```python
from build123d import *

# Parameters (mm, degrees)
SKETCH1_W           = 10
SKETCH1_H           = 7
BOSS_EXTRUDE1_DEPTH = 2
SKETCH2_R           = 1.425
CUT_EXTRUDE1_DEPTH  = 2
SKETCH3_W           = 6
SKETCH3_H           = 1
BOSS_EXTRUDE2_DEPTH = 6


with BuildPart() as part:
    # Sketch1 → Boss-Extrude1 (new body)
    with BuildSketch(Plane(origin=(0, 0, 0), x_dir=(1, 0, 0), z_dir=(0, 1, 0))):
        Rectangle(SKETCH1_W, SKETCH1_H)
    extrude(amount=BOSS_EXTRUDE1_DEPTH)

    # Sketch2 → Cut-Extrude1 (cut)
    with BuildSketch(Plane(origin=(0, 2, 0), x_dir=(1, 0, 0), z_dir=(0, 1, 0))):
        Circle(SKETCH2_R)
    extrude(amount=-CUT_EXTRUDE1_DEPTH, mode=Mode.SUBTRACT)

    # Sketch3 → Boss-Extrude2 (add)
    with BuildSketch(Plane(origin=(0, 2, 0), x_dir=(1, 0, 0), z_dir=(0, 1, 0))):
        with Locations((0, -3)):
            Rectangle(SKETCH3_W, SKETCH3_H)
    boss_extrude2 = extrude(amount=BOSS_EXTRUDE2_DEPTH)

    # Mirror1: Boss-Extrude2 across plane
    add(boss_extrude2.mirror(Plane.XY))


solid = part.part
```
The listing builds one solid part. Answer for the finished solid, in the listing's coordinates (mm). A direction names the side the tool comes from. Give positions to 0.01 mm unless a question says otherwise; leave off trailing zeros. Order: outer loops, then holes, each group sorted by start corner. A loop starts at its lowest first (then second) coordinate and runs counter-clockwise, first axis right, second up.
Item 1: Given pin 1 Ø1.1 at (y, z) = (5.5, -3) entering from -X; pin 2 Ø2 at (y, z) = (5, 0.5) entering from +X, each flat-ended and moving along its own axis, determine where each tip first touches the part or whether it passes through.
From the geometry:
pin 1: stops at x = -3
pin 2: passes through
Item 2: For a pull along Z with two mould halves and no side action, classify faces 1 (the face through (0, 3, 3.5)), 2 (the face through (0, 5, -2.5)), 3 (the face through (0, 8, -3)) as pulls with the +Z half, pulls with the -Z half, needs draft (parallel to the pull), parting line crosses it, or undercut.
From the geometry:
face 1: pulls with the +Z half
face 2: undercut
face 3: needs draft
Item 3: The part is cut by section D-D, the plane y = 1.5. Give the vertices of the cut face in (x, z) (3 decimals).
From the geometry:
outline: (-5, -3.5) - (5, -3.5) - (5, 3.5) - (-5, 3.5) - close; hole circle Ø2.85 at (0, 0)
Item 4: Find the intervals of material crossed by probe 1 along Z at (x, y) = (0, 1.35) (3 decimals); probe 2 along X at (y, z) = (1.5, 0) (3 decimals); probe 3 along Z at (x, y) = (0, 5), in increasing order.
From the geometry:
probe 1: z = -3.5 to -1.425, 1.425 to 3.5
probe 2: x = -5 to -1.425, 1.425 to 5
probe 3: z = -3.5 to -2.5, 2.5 to 3.5
Item 5: Which of the six approach directions +Z, -Z, +X, -X, +Y, -Y give full straight-line access (tool end or side, diameter ignored) to faces 4 (the face through (-3, 5, 3)), 5 (the face through (0, 3, -3.5)), 6 (the face through (0, 5, 2.5)), 7 (the face through (3, 5, -3)), 8 (the face through (0, 8, 3))?
From the geometry:
face 4: +Z, -Z, -X, +Y
face 5: -Z, +X, -X, +Y, -Y
face 6: +X, -X, +Y
face 7: +Z, -Z, +X, +Y
face 8: +Z, -Z, +X, -X, +Y
Item 6: The part is cut by section A-A, the plane y = 5.25. Give the vertices of the cut face in (x, z).
From the geometry:
outline: (-3, -3.5) - (3, -3.5) - (3, -2.5) - (-3, -2.5) - close; (-3, 2.5) - (3, 2.5) - (3, 3.5) - (-3, 3.5) - close
Item 7: The part is cut by section C-C, the plane x = 0. Give the vertices of the cut face in (y, z) (3 decimals).
From the geometry:
outline: (0, -3.5) - (8, -3.5) - (8, -2.5) - (2, -2.5) - (2, -1.425) - (0, -1.425) - close; (0, 1.425) - (2, 1.425) - (2, 2.5) - (8, 2.5) - (8, 3.5) - (0, 3.5) - close
Item 8: The part is cut by section B-B, the plane z = 0. Give the vertices of the cut face in (x, y) (3 decimals).
From the geometry:
outline: (-5, 0) - (-1.425, 0) - (-1.425, 2) - (-5, 2) - close; (1.425, 0) - (5, 0) - (5, 2) - (1.425, 2) - close
